Model file for the job. Use its own axes, mm. A direction names the side the tool comes from. Round coordinates to 2 decimals unless told otherwise and drop trailing zeros. Loops run counter-clockwise (first coordinate to the right, second up) from the corner with the lowest first, then second, coordinate; pieces in that order, holes last.
from build123d import *

# Parameters (mm, degrees)
PAD_DEPTH    = 5
CHAMFER_SIZE = 2


with BuildPart() as part:
    # Sketch → Pad (new body)
    with BuildSketch(Plane.XY):
        with BuildLine():
            ThreePointArc((6.427935, -0.965218), (-2.949616, 5.792216), (-3, -5.766281))
            Line((-3, -5.766281), (-3, -7.066281))
            Line((-3, -7.066281), (-6, -7.066281))
            Line((-6, -7.066281), (-6, -9.066281))
            Line((-6, -9.066281), (6, -9.066281))
            Line((6, -9.066281), (6, -7.066281))
            Line((6, -7.066281), (3, -7.066281))
            Line((3, -7.066281), (3, -5.766281))
            ThreePointArc((3, -5.766281), (3.434671, -5.518427), (3.848989, -5.23787))
            Line((3.848989, -5.23787), (2.664685, -3.626218))
            ThreePointArc((3.972861, -2.113381), (-3.403883, 2.943396), (2.664685, -3.626218))
            Line((3.972861, -2.113381), (7.928513, -2.707361))
            Line((7.928513, -2.707361), (8.151256, -1.223992))
            Line((8.151256, -1.223992), (6.427935, -0.965218))
        make_face()
    extrude(amount=PAD_DEPTH)

    # Chamfer
    chamfer_edges = [part.edges().sort_by_distance(p)[0] for p in [
        (6, -8.066281, 5),
        (3, -6.416281, 5),
        (-3, -6.416281, 0),
        (-6, -8.066281, 0),
    ]]
    chamfer(chamfer_edges, length=CHAMFER_SIZE)


solid = part.part
Q1. Flat gauge pins, fed straight in: P1, Ø2.5, axis at x = -2.5, z = 1.5, coming from the +Y side; P2, Ø1.5, axis at x = 3, z = 3.5, coming from the +Y side; P3, Ø1, axis at y = -8, z = 1.5, coming from the +X side. Where does each tip first touch, or does it go through?
Q2. Tool access for faces 5 (the face through (-4, -7.066, 2)), 6 (the face through (3, -6, 1)), 7 (the face through (4, -7.066, 2)), 8 (the face through (-5, -8, 1)): list every direction of +Z, -Z, +X, -X, +Y, -Y with a clear straight run to the whole face (end or side of a thin tool).
Q3. Slice it at A-A on x = 0. Give the cut face in (y, z), plus the area to 3 significant figures.
Q4. Slice it at D-D on y = -8. Give the cut face in (x, z), plus the area to 3 significant figures.
Q5. Slice it at C-C on z = 2.45. Give the cut face in (x, y), plus the area to 3 significant figures.
Q6. Pull direction X, two halves, no side cores. Call faces 1 (the face through (-2, -6.6, 1)), 2 (the face through (5, -8, 4)), 3 (the face through (-3.28, 3.08, 2.46)), 4 (the face through (-3.674, 5.362, 2.465)): pulls with the +X half, pulls with the -X half, needs draft (parallel to the pull), parting line crosses it, or undercut.
Q7. Slice it at B-B on y = 0. Give the cut face in (x, z), plus the area to 3 significant figures.
Q8. Probe line 1 (X direction, y = 0, z = 1.4); line 2 (Y direction, x = 0, z = 3.9); line 3 (Y direction, x = -3, z = 1.4). List the from-to ranges inside material, lowest first.
Reply:
1. P1: stops at y = 6.38
1. P2: stops at y = 6.1
1. P3: stops at x = 6
2. face 5: -Z, -X
2. face 6: +Z, -Z, +X
2. face 7: +Z, +X
2. face 8: -Z, -X, -Y
3. outline: (-9.07, 0) - (-4.5, 0) - (-4.5, 5) - (-9.07, 5) - close; (4.5, 0) - (6.5, 0) - (6.5, 5) - (4.5, 5) - close
3. area: 32.8 mm2
4. outline: (-6, 2) - (-4, 0) - (6, 0) - (6, 3) - (4, 5) - (-6, 5) - close
4. area: 56.0 mm2
5. outline: (-6, -9.07) - (6, -9.07) - (6, -7.07) - (3, -7.07) - (3, -5.77) arc R6.5 ccw to (3.85, -5.24) - (2.66, -3.63) arc R4.5 cw (long way) to (3.97, -2.11) - (7.93, -2.71) - (8.15, -1.22) - (6.43, -0.97) arc R6.5 ccw (long way) to (-3, -5.77) - (-3, -7.07) - (-6, -7.07) - close
5. area: 95.0 mm2
6. face 1: pulls with the -X half
6. face 2: pulls with the +X half
6. face 3: undercut
6. face 4: parting line crosses it
7. outline: (-6.5, 0) - (-4.5, 0) - (-4.5, 5) - (-6.5, 5) - close; (4.5, 0) - (6.5, 0) - (6.5, 5) - (4.5, 5) - close
7. area: 20.0 mm2
8. line 1: x = -6.5 to -4.5, 4.5 to 6.5
8. line 2: y = -9.07 to -4.5, 4.5 to 6.5
8. line 3: y = -9.07 to -7.07, -5.77 to -3.35, 3.35 to 5.77
